Source: three-view drawing plus pictorial views. Frame: mm from the lowest corner of the part. A direction names the side the tool comes from. Give positions to 0.01 mm unless a question says otherwise; leave off trailing zeros. Order: outer loops, then holes, each group sorted by start corner. A loop starts at its lowest first (then second) coordinate and runs counter-clockwise, first axis right, second up.
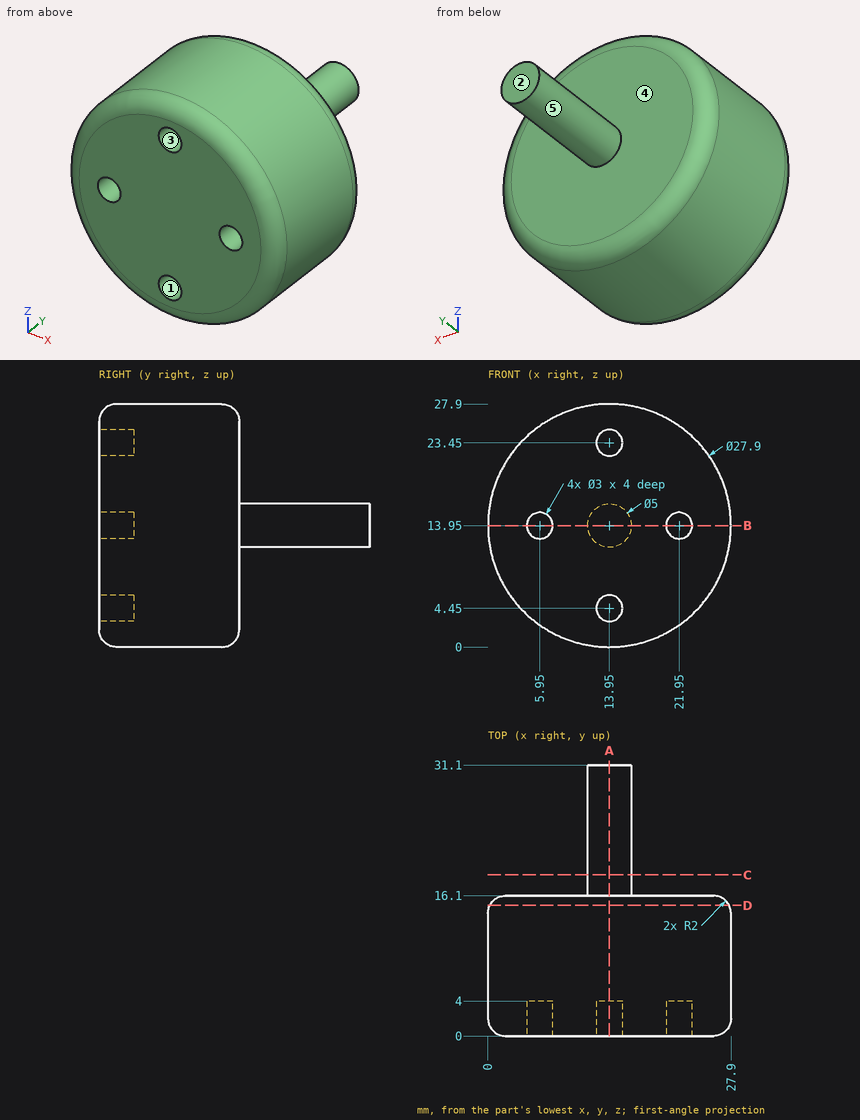
1) Section query B-B on z = 13.95. Output: boundary loops of the cut face in (x, y).
Checks:
outline: (0, 2) arc R2 ccw to (2, 0) - (4.45, 0) - (4.45, 4) - (7.45, 4) - (7.45, 0) - (20.45, 0) - (20.45, 4) - (23.45, 4) - (23.45, 0) - (25.9, 0) arc R2 ccw to (27.9, 2) - (27.9, 14.1) arc R2 ccw to (25.9, 16.1) - (16.45, 16.1) - (16.45, 31.1) - (11.45, 31.1) - (11.45, 16.1) - (2, 16.1) arc R2 ccw to (0, 14.1) - close
2) Pull-direction query (X, two-part tool) for the marked faces 3, 4 and 5; classes: +X half, -X half, draft (parallel to the pull), parting line (faces both ways), or undercut.
Checks:
face 3: undercut
face 4: draft
face 5: parting line
3) Ray query, L1, parallel to Z at x = 13.95, y = 2.1; L2, parallel to Y at x = 19, z = 21; L3, parallel to Z at x = 5.95, y = 3.05. Return the intervals inside material, ascending.
Checks:
L1: z = 0 to 2.95, 5.95 to 21.95, 24.95 to 27.9
L2: y = 0 to 16.1
L3: z = 2.52 to 12.45, 15.45 to 25.38
4) Section query D-D on y = 15. Output: boundary loops of the cut face in (x, z), and give its area (3 significant figures).
Checks:
outline: circle Ø27.47 at (13.95, 13.95)
area: 593 mm2
5) Section query A-A on x = 13.95. Output: boundary loops of the cut face in (y, z).
Checks:
outline: (0, 2) arc R2 ccw to (2, 0) - (14.1, 0) arc R2 ccw to (16.1, 2) - (16.1, 11.45) - (31.1, 11.45) - (31.1, 16.45) - (16.1, 16.45) - (16.1, 25.9) arc R2 ccw to (14.1, 27.9) - (2, 27.9) arc R2 ccw to (0, 25.9) - (0, 24.95) - (4, 24.95) - (4, 21.95) - (0, 21.95) - (0, 5.95) - (4, 5.95) - (4, 2.95) - (0, 2.95) - close
6) First-contact query: pin 1 Ø3 at (x, z) = (14, 20) entering from +Y; pin 2 Ø1.5 at (x, z) = (14, 5) entering from -Y; pin 3 Ø12 at (y, z) = (10.5, 25) entering from -X. Flat tips, straight axial feed; report the tip coordinate or a pass-through.
Checks:
pin 1: stops at y = 16.1
pin 2: stops at y = 4
pin 3: stops at x = 0.95
7) Section query C-C on y = 18.5. Output: boundary loops of the cut face in (x, z), and give its area (3 significant figures).
Checks:
outline: circle Ø5 at (13.95, 13.95)
area: 19.6 mm2
8) Reachability of the marked faces 1 and 2 from +Z, -Z, +X, -X, +Y, -Y: full face, straight path, thin tool, end or side. Return the list, or none.
Checks:
face 1: -Y
face 2: +Z, -Z, +X, -X, +Y
